Could you check a few things on this model? Use its own coordinates, in mm. A direction names the side the tool comes from. Give positions to 0.01 mm unless a question says otherwise; leave off trailing zeros. Loops run counter-clockwise (first coordinate to the right, second up) from the corner with the lowest first, then second, coordinate; pieces in that order, holes last. Notation, with made-up numbers: M 34.25,72 L 74.25,72 A34 ccw 74.25,102 Z; hole C -10.75,47 d2. An arc over 180 degrees is marked long. Return JSON: item names as keys, results as strings. Group by question number.
1. If we section it at B-B (x = 30): Write out the boundary of the cut face in (y, z), plus the area to 3 significant figures.
2. For pin 1 (4 mm diameter, centred on y = -0.5, z = -15, fed in from +X); pin 2 (2 mm diameter, centred on x = -25.5, y = 1, fed in from -Z); pin 3 (1.5 mm diameter, centred on x = -8, z = -3.5, fed in from +Y); pin 4 (1.6 mm diameter, centred on x = -26, y = 1, fed in from -Z), each with a flat end and sliding along its axis, tell me the tip position at first contact or that it passes through.
3. Please list where these lines run through material, in increasing order: line 1 (Z direction, x = 0, y = 0.5); line 2 (Z direction, x = 4.5, y = 3); line 3 (X direction, y = 1, z = 10).
4. If we mould it in two halves opening along X, with no side actions, what happens to faces 1 (the cylindrical face through (13.036, -0.053, 7.421)), 2 (the flat face through (-30.08, -0.05, -12.98)), 3 (the flat face through (-28.019, -0.053, -8.265))? For each: +X half, -X half, draft (parallel to the pull), parting line (faces both ways), or undercut.
5. If we section it at C-C (y = 0): State how many separate pieces and enclosed holes the cut face has, plus the area to 3 significant figures.
6. If we section it at A-A (z = 0): Write out the boundary of the cut face in (x, y), plus the area to 3 significant figures.
7. For faces 4 (the flat face through (3.415, 0.053, 34.612)), 5 (the flat face through (-6.3, 3.75, -9.4)), 6 (the flat face through (21.167, -0.053, -20.133)), which set-ups out of +Z, -Z, +X, -X, +Y, -Y let a thin tool reach every point of the face, with its end or its side?
```python
from build123d import *

# Parameters (mm, degrees)
F0_R     = 10.9
F1_DEPTH = 3.75


with BuildPart() as f1:
    # F0 (on Front) → F1 (new body, symmetric)
    with BuildSketch(Plane.XZ):
        with BuildLine():
            ThreePointArc((14.937581, 1.366992), (14.984387, 0.684208), (15, 0))
            ThreePointArc((15, 0), (12.634756, -8.084735), (6.284941, -13.619821))
            Line((6.284941, -13.619821), (36.471143, -26.830127))
            Line((36.471143, -26.830127), (38.971143, -22.5))
            Line((38.971143, -22.5), (41.471143, -18.169873))
            Line((41.471143, -18.169873), (14.937581, 1.366992))
        make_face()
        Polygon((31.738434, -17.805939), (27.021887, -20.839044), (22.036867, -18.270946), (21.768395, -12.669745), (26.484942, -9.63664), (31.469961, -12.204737), align=None, mode=Mode.SUBTRACT)
        with BuildLine():
            Line((-36.471143, -26.830127), (-6.284941, -13.619821))
            ThreePointArc((-6.284941, -13.619821), (-12.990381, -7.5), (-14.937581, 1.366992))
            Line((-14.937581, 1.366992), (-41.471143, -18.169873))
            Line((-41.471143, -18.169873), (-38.971143, -22.5))
            Line((-38.971143, -22.5), (-36.471143, -26.830127))
        make_face()
        Polygon((-31.384168, -15.239825), (-28.740776, -10.661338), (-23.453994, -10.661338), (-20.810603, -15.239825), (-23.453994, -19.818313), (-28.740776, -19.818313), align=None, mode=Mode.SUBTRACT)
        with BuildLine():
            ThreePointArc((-8.65264, 12.252829), (0, 15), (8.65264, 12.252829))
            Line((8.65264, 12.252829), (5, 45))
            Line((5, 45), (0, 45))
            Line((0, 45), (-5, 45))
            Line((-5, 45), (-8.65264, 12.252829))
        make_face()
        Polygon((4.037737, 33.466694), (5.380126, 31.273188), (5.305265, 31.135505), (5.380126, 30.997823), (4.037737, 28.804316), (2.8093, 26.54502), (2.652632, 26.541011), (2.570827, 26.407338), (0, 26.473128), (-2.570827, 26.407338), (-2.652632, 26.541011), (-2.8093, 26.54502), (-4.037737, 28.804316), (-5.380126, 31.273188), (-2.570827, 35.863672), (2.652632, 35.729999), (2.8093, 35.72599), align=None, mode=Mode.SUBTRACT)
        Circle(F0_R)
        with BuildLine():
            ThreePointArc((6.284941, -13.619821), (12.634756, -8.084735), (15, 0))
            ThreePointArc((15, 0), (14.984387, 0.684208), (14.937581, 1.366992))
            ThreePointArc((14.937581, 1.366992), (12.990381, 7.5), (8.65264, 12.252829))
            ThreePointArc((8.65264, 12.252829), (0, 15), (-8.65264, 12.252829))
            ThreePointArc((-8.65264, 12.252829), (-12.990381, 7.5), (-14.937581, 1.366992))
            ThreePointArc((-14.937581, 1.366992), (-12.990381, -7.5), (-6.284941, -13.619821))
            ThreePointArc((-6.284941, -13.619821), (0, -15), (6.284941, -13.619821))
        make_face()
        Circle(F0_R, mode=Mode.SUBTRACT)
    extrude(amount=F1_DEPTH, both=True)


solid = f1.part
```
Answer:
{
 "1": {"outline": "M -3.75,-24 L 3.75,-24 L 3.75,-18.92 L -3.75,-18.92 Z; M -3.75,-11.45 L 3.75,-11.45 L 3.75,-9.72 L -3.75,-9.72 Z", "area": "51.0 mm²"},
 "2": {"pin 1": "stops at x = 39.88", "pin 2": "stops at z = -22.47", "pin 3": "passes through", "pin 4": "stops at z = -22.6"},
 "3": {"line 1": "z = -15 to -10.9, 10.9 to 26.47, 35.8 to 45", "line 2": "z = -14.31 to -9.93, 9.93 to 29.56, 32.71 to 45", "line 3": "x = -11.18 to -4.34, 4.34 to 11.18"},
 "4": {"face 1": "+X half", "face 2": "undercut", "face 3": "-X half"},
 "5": {"separate pieces": "1", "enclosed holes": "4", "area": "1,350 mm²"},
 "6": {"outline": "M -16.79,-3.75 L -10.9,-3.75 L -10.9,3.75 L -16.79,3.75 Z; M 10.9,-3.75 L 16.79,-3.75 L 16.79,3.75 L 10.9,3.75 Z", "area": "88.4 mm²"},
 "7": {"face 4": "+Y, -Y", "face 5": "+Z, -Z, +X, -X, +Y", "face 6": "-Z, +Y, -Y"}
}
